```python
from build123d import *

# Parameters (mm, degrees)
EXTRUDE1_DEPTH      = 10
EXTRUDE2_DEPTH      = 10
EXTRUDE3_DEPTH      = 10
SKETCH2_W           = 9.998469457
SKETCH2_H           = 10.103213958
SKETCH2_W_2         = 10.103213958
SKETCH2_W_3         = 10.643545952
SKETCH2_W_4         = 9.998494457
EXTRUDE4_DEPTH      = 10
EXTRUDE4_DEPTH_BACK = 99


with BuildPart() as part:
    # Sketch1 → Extrude1 (new body)
    with BuildSketch(Plane.XY):
        Polygon((63.686330841, 43.028866588), (73.609130264, 43.028866588), (114.021986095, 43.028866588), (114.021986095, 53.132080546), (-114.021986095, 53.132080546), (-114.021986095, 43.028866588), (-73.609130264, 43.028866588), (-63.505916306, 43.028866588), align=None)
    extrude(amount=EXTRUDE1_DEPTH)



with BuildPart() as body_2:
    # Sketch1<3> → Extrude2 (new body)
    with BuildSketch(Plane.XY):
        Polygon((40.232441296, -51.869178801), (40.232441296, -41.765964843), (30.129227338, -41.765964843), (-29.768398268, -41.765964843), (-39.871612226, -41.765964843), (-39.871612226, -51.869178801), align=None)
    extrude(amount=EXTRUDE2_DEPTH)


with BuildPart() as part_1:
    add(part.part)

    add(body_2.part)  # Extrude3 merges body 2
    # Sketch1<4> → Extrude3 (add)
    with BuildSketch(Plane.XY):
        Polygon((40.232441296, -41.765964843), (73.609130264, 43.028866588), (63.686330841, 43.028866588), (30.129227338, -41.765964843), align=None)
        Polygon((-29.768398268, -41.765964843), (-63.505916306, 43.028866588), (-73.609130264, 43.028866588), (-39.871612226, -41.765964843), align=None)
    extrude(amount=EXTRUDE3_DEPTH)

    # Sketch2 → Extrude4 (add, two sides)
    with BuildSketch(Plane.XY) as extrude4_sk:
        with Locations((-109.022751367, 48.080473567)):
            Rectangle(SKETCH2_W, SKETCH2_H)
        with Locations((-34.820005247, -46.817571822)):
            Rectangle(SKETCH2_W_2, SKETCH2_H)
        with Locations((34.91066832, -46.817571822)):
            Rectangle(SKETCH2_W_3, SKETCH2_H)
        with Locations((109.022738867, 48.080473567)):
            Rectangle(SKETCH2_W_4, SKETCH2_H)
    extrude(amount=EXTRUDE4_DEPTH)
    extrude(extrude4_sk.sketch, amount=-EXTRUDE4_DEPTH_BACK)


solid = part_1.part
```
CAD build for the part. Positions are in the model's coordinates, mm. A direction names the side the tool comes from. Give positions to 0.01 mm unless a question says otherwise; leave off trailing zeros. Loops run counter-clockwise (first coordinate to the right, second up) from the corner with the lowest first, then second, coordinate; pieces in that order, holes last. Notation, with made-up numbers: (17.25, -12.5) -> (66.25, -12.5) arc R21 cw to (66.25, 21.5) -> close; hole circle Ø11 at (84, 42.5). An arc over 180 degrees is marked (long way). Use a Markdown table: item, result.
1. Slice it at C-C (y = 31). List the corners of the cut face in (x, z), plus the area to 3 significant figures.
Check result:
| item | result |
|---|---|
| outline | (-68.82, 0) -> (-58.72, 0) -> (-58.72, 10) -> (-68.82, 10) -> close; (58.93, 0) -> (68.87, 0) -> (68.87, 10) -> (58.93, 10) -> close |
| area | 201 mm^2 |
2. Slice it at B-B (z = 3). List the corners of the cut face in (x, y).
Check result:
| item | result |
|---|---|
| outline | (-114.02, 43.03) -> (-73.61, 43.03) -> (-39.87, -41.77) -> (-39.87, -51.87) -> (40.23, -51.87) -> (40.23, -41.77) -> (73.61, 43.03) -> (114.02, 43.03) -> (114.02, 53.13) -> (-114.02, 53.13) -> close; hole (-63.51, 43.03) -> (-29.77, -41.77) -> (30.13, -41.77) -> (63.69, 43.03) -> close |
3. Flat gauge pins, fed straight in: pin 1 (10 mm diameter, centred on x = -32, z = -62, fed in from +Y); pin 2 (3 mm diameter, centred on x = 14.5, y = -47.5, fed in from -Z); pin 3 (20 mm diameter, centred on x = -97.5, z = -26.5, fed in from -Y). Where does each tip first touch, or does it go through?
Check result:
| item | result |
|---|---|
| pin 1 | stops at y = -41.77 |
| pin 2 | stops at z = 0 |
| pin 3 | stops at y = 43.03 |
4. Slice it at A-A (x = 13.5). List the corners of the cut face in (y, z), plus the area to 3 significant figures.
Check result:
| item | result |
|---|---|
| outline | (-51.87, 0) -> (-41.77, 0) -> (-41.77, 10) -> (-51.87, 10) -> close; (43.03, 0) -> (53.13, 0) -> (53.13, 10) -> (43.03, 10) -> close |
| area | 202 mm^2 |
5. Slice it at D-D (z = -12). List the corners of the cut face in (x, y).
Check result:
| item | result |
|---|---|
| outline | (-114.02, 43.03) -> (-104.02, 43.03) -> (-104.02, 53.13) -> (-114.02, 53.13) -> close; (-39.87, -51.87) -> (-29.77, -51.87) -> (-29.77, -41.77) -> (-39.87, -41.77) -> close; (29.59, -51.87) -> (40.23, -51.87) -> (40.23, -41.77) -> (29.59, -41.77) -> close; (104.02, 43.03) -> (114.02, 43.03) -> (114.02, 53.13) -> (104.02, 53.13) -> close |
6. Which spindle directions (+Z, -Z, +X, -X, +Y, -Y) get a long thin tool onto all of the face, cutting with end or side? Do faces 5 (the flat face through (-35, -41.766, -49)), 6 (the flat face through (31, -41.766, -33)), 7 (the flat face through (29.589, -47, -49)), 8 (the flat face through (47.143, 1.225, 4.93)). Say none if no direction does.
Check result:
| item | result |
|---|---|
| face 5 | -Z, +X, -X, +Y |
| face 6 | -Z |
| face 7 | -Z, +Y, -Y |
| face 8 | +Z, -Z |
7. Mould opens along X. For faces 1 (the flat face through (-1, -47, 0)), 2 (the flat face through (56.69, 0.04, 4.93)), 3 (the flat face through (-114.022, 48, -44)), 4 (the flat face through (-35, -47, -99)) say: pulls with the +X half, pulls with the -X half, needs draft (parallel to the pull), parting line crosses it, or undercut.
Check result:
| item | result |
|---|---|
| face 1 | undercut |
| face 2 | pulls with the +X half |
| face 3 | pulls with the -X half |
| face 4 | needs draft |
8. Wall check: L1, parallel to X at y = 45.5, z = -0.5; L2, parallel to Z at x = -61, y = 47; L3, parallel to X at y = -46, z = -9.5. Give the ranges that are in metal, low to high. Write a range as [from, to].
Check result:
| item | result |
|---|---|
| L1 | x = [-114.02, -104.02], [104.02, 114.02] |
| L2 | z = [0, 10] |
| L3 | x = [-39.87, -29.77], [29.59, 40.23] |
